from build123d import *

# Parameters (mm, degrees)
SKETCH_1_W          = 70
SKETCH_1_H          = 30
EXTRUDE_1_DEPTH     = 5
SKETCH_2_R          = 3.15
CUT_EXTRUDE_1_DEPTH = 5
SKETCH_3_W          = 30
SKETCH_3_H          = 30
EXTRUDE_2_DEPTH     = 35
SKETCH_4_R          = 9.7
CUT_EXTRUDE_2_DEPTH = 30
CHAMFER_1_SIZE      = 5
SKETCH_5_W          = 4
SKETCH_5_H          = 18
CUT_EXTRUDE_3_DEPTH = 30
FILLET_1_R          = 5
SKETCH_6_R          = 3.2
CUT_EXTRUDE_4_DEPTH = 30
SKETCH_7_R          = 6
CUT_EXTRUDE_5_DEPTH = 6
CUT_EXTRUDE_6_DEPTH = 6
FILLET_2_R          = 5
CHAMFER_2_SIZE      = 2


with BuildPart() as part:
    # 草图1 → 凸台-拉伸1 (new body)
    with BuildSketch(Plane.XY):
        Rectangle(SKETCH_1_W, SKETCH_1_H)
    extrude(amount=EXTRUDE_1_DEPTH)

    # 草图2 → 切除-拉伸1 (cut)
    with BuildSketch(Plane.XY.offset(5)):
        with Locations((-25, 0)):
            Circle(SKETCH_2_R)
        with Locations((25, 0)):
            Circle(SKETCH_2_R)
    extrude(amount=-CUT_EXTRUDE_1_DEPTH, mode=Mode.SUBTRACT)

    # 草图3 → 凸台-拉伸2 (add)
    with BuildSketch(Plane.XY.offset(5)):
        Rectangle(SKETCH_3_W, SKETCH_3_H)
    extrude(amount=EXTRUDE_2_DEPTH)

    # 草图4 → 切除-拉伸2 (cut)
    with BuildSketch(Plane(origin=(0, 15, 0), x_dir=(1, 0, 0), z_dir=(0, 1, 0))):
        with Locations(Location((0, -16, 0), (0, 0, 270))):
            Circle(SKETCH_4_R)
    extrude(amount=-CUT_EXTRUDE_2_DEPTH, mode=Mode.SUBTRACT)

    # 倒角1
    chamfer_1_edges = [part.edges().sort_by_distance(p)[0] for p in [
        (0, -15, 6.3),
    ]]
    chamfer(chamfer_1_edges, length=CHAMFER_1_SIZE)

    # 草图5 → 切除-拉伸3 (cut)
    with BuildSketch(Plane(origin=(0, 15, 0), x_dir=(1, 0, 0), z_dir=(0, 1, 0))):
        with Locations((0, -31)):
            Rectangle(SKETCH_5_W, SKETCH_5_H)
    extrude(amount=-CUT_EXTRUDE_3_DEPTH, mode=Mode.SUBTRACT)

    # 圆角1
    fillet_1_edges = [part.edges().sort_by_distance(p)[0] for p in [
        (2, 2.5, 25.491575212),
        (-2, 2.5, 25.491575212),
    ]]
    fillet(fillet_1_edges, radius=FILLET_1_R)

    # 草图6 → 切除-拉伸4 (cut)
    with BuildSketch(Plane(origin=(15, 0, 0), x_dir=(0, 0, -1), z_dir=(1, 0, 0))):
        with Locations(Location((-33, 0, 0), (0, 0, 90))):
            Circle(SKETCH_6_R)
    extrude(amount=-CUT_EXTRUDE_4_DEPTH, mode=Mode.SUBTRACT)

    # 草图7 → 切除-拉伸5 (cut)
    with BuildSketch(Plane(origin=(15, 0, 0), x_dir=(0, 0, -1), z_dir=(1, 0, 0))):
        with Locations(Location((-33, 0, 0), (0, 0, 90))):
            Circle(SKETCH_7_R)
    extrude(amount=-CUT_EXTRUDE_5_DEPTH, mode=Mode.SUBTRACT)

    # 草图8 → 切除-拉伸6 (cut)
    with BuildSketch(Plane.ZY.offset(15)):
        Polygon((28, -2.886751346), (33, -5.773502692), (38, -2.886751346), (38, 2.886751346), (33, 5.773502692), (28, 2.886751346), align=None)
    extrude(amount=-CUT_EXTRUDE_6_DEPTH, mode=Mode.SUBTRACT)

    # 圆角2
    # the kernel refuses this fillet: 5 mm, written as the material it takes off along each edge
    with BuildSketch(Plane(origin=(-15, -27.5, 40), x_dir=(1, 0, 0), z_dir=(0, 1, 0)), Plane(origin=(15, 27.5, 40), x_dir=(-1, 0, 0), z_dir=(0, -1, 0))) as fillet_2_piece_1:
        with BuildLine():
            CenterArc((FILLET_2_R, FILLET_2_R), FILLET_2_R, 180, 90)
            Line((0, FILLET_2_R), (0, 0))
            Line((0, 0), (FILLET_2_R, 0))
        make_face()
    extrude(amount=55, mode=Mode.SUBTRACT)

    # 倒角2
    chamfer_2_edges = [part.edges().sort_by_distance(p)[0] for p in [
        (2, 15, 34.463164859),
        (0, 15, 6.3),
        (-2, 15, 34.463164859),
        (-2.704376535, 15, 26.36749814),
        (2.704376535, 15, 26.36749814),
    ]]
    chamfer(chamfer_2_edges, length=CHAMFER_2_SIZE)


solid = part.part
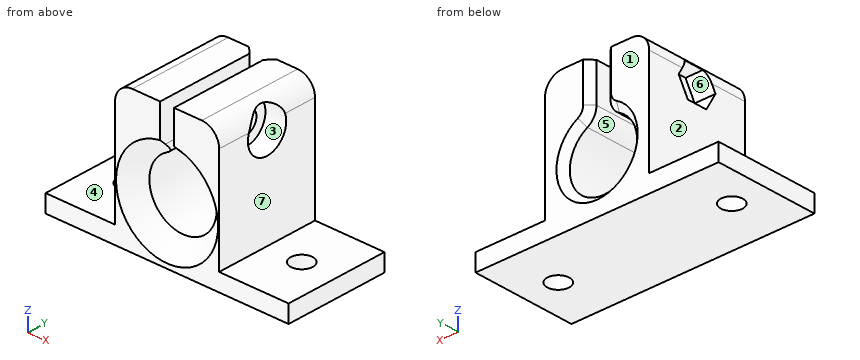
CAD build for the part. Positions are in the model's coordinates, mm. Face numbers are marked on the shaded views. A direction names the side the tool comes from. Round coordinates to 2 decimals unless told otherwise and drop trailing zeros. Order: outer loops, then holes, each group sorted by start corner. A loop starts at its lowest first (then second) coordinate and runs counter-clockwise, first axis right, second up. Notation, with made-up numbers: (72, 43) -> (99, 43) arc R6 cw to (99, 49) -> close; hole circle Ø10 at (-11.5, 13.25). An arc over 180 degrees is marked (long way). Write item = value, one per line. Start each with the question number.
(1) Pin check, flat tips, straight feed: P1, Ø1, axis at y = 9.5, z = 10.5, coming from the -X side; P2, Ø8, axis at x = 6.5, z = 11, coming from the -Y side; P3, Ø16, axis at x = -25.5, y = 5, coming from the +Z side. Stop position of each tip, or through.
(2) Probe line 1 (X direction, y = 8.5, z = 16); line 2 (Z direction, x = -2.5, y = 2); line 3 (X direction, y = 13, z = 32). List the from-to ranges inside material, lowest first. Write a range as [from, to].
(3) Pull direction Y, two halves, no side cores. Call the marked faces 1, 2 and 3: released by +Y, released by -Y, zero draft, split by the parting line, or undercut.
(4) Cut at D-D, the plane x = 16.5. List the corners of the cut face in (y, z).
(5) Cut at A-A, the plane z = 16. List the corners of the cut face in (x, y), then the cut area to 3 significant figures.
(6) Cut at C-C, the plane y = 0. State how many separate pieces and enclosed holes the cut face has, then the cut area to 3 significant figures.
(7) Cut at B-B, the plane x = -25. List the corners of the cut face in (y, z), then the cut area to 4 significant figures.
(8) Which spindle directions (+Z, -Z, +X, -X, +Y, -Y) get a long thin tool onto all of the face, cutting with end or side? Do the marked faces 4, 5, 6 and 7. Say none if no direction does.
Model answer:
q1.P1 = -15
q1.P2 = -12.5
q1.P3 = 5
q2.line_1 = [-15, -9.7], [9.7, 15]
q2.line_2 = [0, 6.63], [26.75, 30.5], [35.5, 40]
q2.line_3 = [-15, -2], [2, 15]
q3.face_1 = released by +Y
q3.face_2 = zero draft
q3.face_3 = undercut
q4.outline = (-15, 0) -> (15, 0) -> (15, 5) -> (-15, 5) -> close
q5.outline = (-15, -15) -> (-14.7, -15) -> (-9.7, -10) -> (-9.7, 13) -> (-11.7, 15) -> (-15, 15) -> close; (9.7, -10) -> (14.7, -15) -> (15, -15) -> (15, 15) -> (11.7, 15) -> (9.7, 13) -> close
q5.area = 289 mm2
q6.separate_pieces = 5
q6.enclosed_holes = 0
q6.area = 751 mm2
q7.outline = (-15, 0) -> (-3.15, 0) -> (-3.15, 5) -> (-15, 5) -> close; (3.15, 0) -> (15, 0) -> (15, 5) -> (3.15, 5) -> close
q7.area = 118.5 mm2
q8.face_4 = +Z, -X, +Y, -Y
q8.face_5 = +Y, -Y
q8.face_6 = -X
q8.face_7 = +Z, +X, +Y, -Y
